Can you work these out from the model? Positions are in its coordinate system, mm. Face numbers are marked on the shaded views. A direction names the side the tool comes from. Give positions to 0.01 mm unless a question says otherwise; leave off trailing zeros. Loops run counter-clockwise (first coordinate to the right, second up) from the corner with the lowest first, then second, coordinate; pieces in that order, holes last. Notation, with made-up numbers: M 29,73 L 68,73 A25 ccw 68,105 Z; hole C 60,46.5 d10. An arc over 180 degrees is marked long. Answer as a JSON object with one key per item and string values.
```python
from build123d import *

# Parameters (mm, degrees)
F1_DEPTH = 10.16
F2_R     = 4.7625
F3_DEPTH = 25.4
F4_SIZE  = 1.27


with BuildPart() as f1:
    # F0 (on Front) → F1 (new body)
    with BuildSketch(Plane.XZ):
        Polygon((7.715837, 2.917203), (1.331547, 8.140713), (-6.38429, 5.22351), (-7.715837, -2.917203), (-1.331547, -8.140713), (6.38429, -5.22351), align=None)
    extrude(amount=-F1_DEPTH)

    # F2 (on Front) → F3 (join)
    with BuildSketch(Plane.XZ):
        Circle(F2_R)
    extrude(amount=F3_DEPTH)

    # F4
    f4_edges = [f1.edges().sort_by_distance(p)[0] for p in [
        (-7.050064, 10.16, 1.153154),
        (-2.526371, 10.16, 6.682111),
        (4.523692, 10.16, 5.528958),
        (-4.523692, 10.16, -5.528958),
        (2.526371, 10.16, -6.682111),
        (7.050064, 10.16, -1.153154),
    ]]
    chamfer(f4_edges, length=F4_SIZE)


solid = f1.part
```
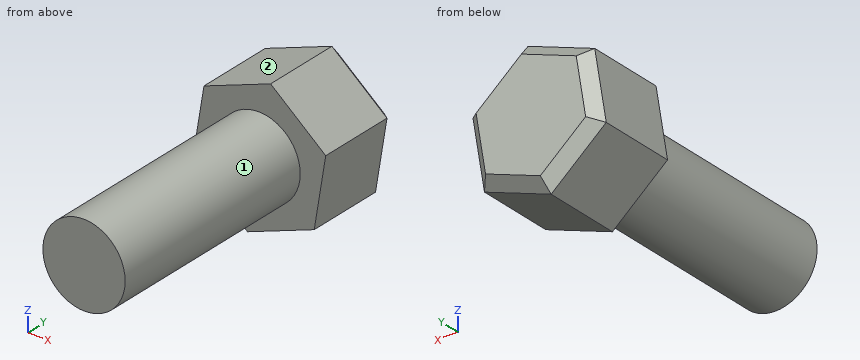
1) Will these pins go through, and if not, where does the flat tip stop? pin 1 Ø1.5 at (y, z) = (-15.5, -3.5) entering from +X; pin 2 Ø6 at (y, z) = (-18, 4) entering from -X; pin 3 Ø3 at (x, y) = (2.5, -16) entering from -Z; pin 4 Ø6 at (x, z) = (-2.5, -6) entering from +Y.
Answer list:
{"pin 1": "x = 3.89", "pin 2": "x = -4.66", "pin 3": "z = -4.66", "pin 4": "y = 10.16"}
2) Suppose I cut it at B-B, the plane x = 0. Write out the boundary of the cut face in (y, z).
Answer list:
{"outline": "M -25.4,-4.76 L 0,-4.76 L 0,-7.64 L 8.89,-7.64 L 10.16,-6.28 L 10.16,6.28 L 8.89,7.64 L 0,7.64 L 0,4.76 L -25.4,4.76 Z"}
3) Suppose I cut it at A-A, the plane z = 0. Write out the boundary of the cut face in (x, y), and give its area (3 significant figures).
Answer list:
{"outline": "M -7.24,0 L -4.76,0 L -4.76,-25.4 L 4.76,-25.4 L 4.76,0 L 7.24,0 L 7.24,8.89 L 5.95,10.16 L -5.95,10.16 L -7.24,8.89 Z", "area": "387 mm^2"}
4) Please list where these lines run through material, in increasing order: line 1 along Y through (x, z) = (-2, 4.75); line 2 along X through (y, z) = (-15.5, 1.75); line 3 along X through (y, z) = (-7, -3.25). Write a range as from..to.
Answer list:
{"line 1": "0..10.16", "line 2": "-4.43..4.43", "line 3": "-3.48..3.48"}
5) Suppose I cut it at D-D, the plane x = 6. Write out the boundary of the cut face in (y, z).
Answer list:
{"outline": "M 0,-5.37 L 8.89,-5.37 L 9.32,-4.91 L 10.16,0.29 L 10.16,2.68 L 8.89,4.32 L 0,4.32 Z"}
6) Suppose I cut it at C-C, the plane y = -20.5. Write out the boundary of the cut face in (x, z) (1 decimal), and give its area (3 significant figures).
Answer list:
{"outline": "C 0,0 d9.5", "area": "71.3 mm^2"}
7) For the marked faces 1 and 2, which set-ups out of +Z, -Z, +X, -X, +Y, -Y let a thin tool reach every point of the face, with its end or its side?
Answer list:
{"face 1": "-Y", "face 2": "+Z, -X, +Y, -Y"}
